Check sheet for the modelled part. Datum: model origin and axes. Units: mm. Face numbers are marked on the shaded views. A direction names the side the tool comes from. Round coordinates to 2 decimals unless told otherwise and drop trailing zeros. Write each loop counter-clockwise with the first axis right and the second up, starting at its lowest first coordinate (ties: lowest second). Pieces come first, ordered by that corner, then holes. Notation, with made-up numbers: (-20.5, 9) -> (26.5, 9) arc R12 cw to (26.5, 32) -> close; hole circle Ø1 at (42.5, 1). An arc over 180 degrees is marked (long way). Put each result on its own line as item: value. Start each with the question number.
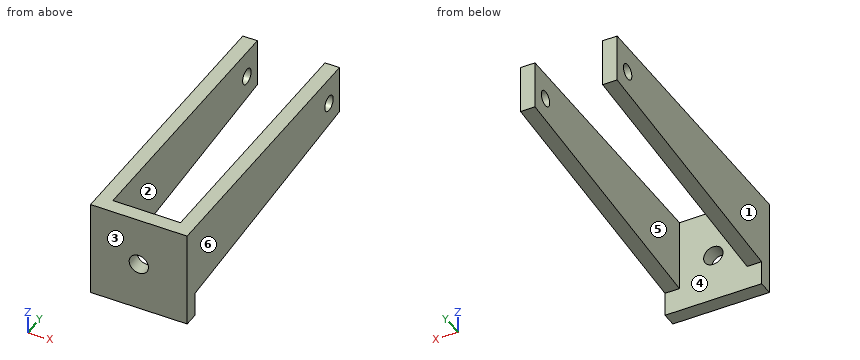
from build123d import *

# Parameters (mm, degrees)
SKETCH_1_W          = 20
SKETCH_1_H          = 20
EXTRUDE_1_DEPTH     = 3
EXTRUDE_2_DEPTH     = 3
EXTRUDE_3_DEPTH     = 3
SKETCH_6_R          = 1.6
CUT_EXTRUDE_1_DEPTH = 21
SKETCH_8_R          = 2
CUT_EXTRUDE_2_DEPTH = 4


with BuildPart() as part:
    # 草图1 → 凸台-拉伸1 (new body)
    with BuildSketch(Plane(origin=(0, 0, 0), x_dir=(1, 0, 0), z_dir=(0, 1, 0))):
        Rectangle(SKETCH_1_W, SKETCH_1_H)
    extrude(amount=EXTRUDE_1_DEPTH)

    # 草图4 → 凸台-拉伸2 (add)
    with BuildSketch(Plane.ZY.offset(10)):
        Polygon((10, 3), (10, 58), (0, 58), (-5, 3), align=None)
    extrude(amount=-EXTRUDE_2_DEPTH)

    # 草图5 → 凸台-拉伸3 (add)
    with BuildSketch(Plane(origin=(10, 0, 0), x_dir=(0, 0, -1), z_dir=(1, 0, 0))):
        Polygon((-10, 3), (5, 3), (0, 58), (-10, 58), align=None)
    extrude(amount=-EXTRUDE_3_DEPTH)

    # 草图6 → 切除-拉伸1 (cut, through all)
    with BuildSketch(Plane(origin=(10, 0, 0), x_dir=(0, 0, -1), z_dir=(1, 0, 0))):
        with Locations((-4.5, 54)):
            Circle(SKETCH_6_R)
    extrude(amount=-CUT_EXTRUDE_1_DEPTH, mode=Mode.SUBTRACT)

    # 草图8 → 切除-拉伸2 (cut, through all)
    with BuildSketch(Plane(origin=(0, 3, 0), x_dir=(1, 0, 0), z_dir=(0, 1, 0))):
        Circle(SKETCH_8_R)
    extrude(amount=-CUT_EXTRUDE_2_DEPTH, mode=Mode.SUBTRACT)


solid = part.part
1. Section check B-B, the plane y = 22.5. Enter the section's corners in (x, z), then the cut area to 3 significant figures.
2. Section check A-A, the plane x = 0. Enter the section's corners in (y, z), then the cut area to 3 significant figures.
3. Draft check along X on the marked faces 3, 4, 5 and 6. Enter one of: released by +X, released by -X, zero draft, split by the parting line, or undercut.
4. Gauge pin test, flat end, axial feed: P1, Ø1.5, axis at x = -1, z = 5, coming from the +Y side. Record the tip position at first contact, or that the pin passes through.
5. Access from +Z, -Z, +X, -X, +Y, -Y to the whole of each face (thin tool, end or side, straight path). Record for the marked faces 1 and 2.
6. Section check D-D, the plane x = -8. Enter the section's corners in (y, z).
7. Section check C-C, the plane z = -3.25. Enter the section's corners in (x, y), then the cut area to 4 significant figures.
8. Material ranges on L1, parallel to X at y = 1, z = 0; L2, parallel to Y at x = 7.6, z = 4.5; L3, parallel to X at y = 45.5, z = 9, recorded low to high. Write a range as [from, to].
Reply:
1. outline: (-10, -3.23) -> (-7, -3.23) -> (-7, 10) -> (-10, 10) -> close; (7, -3.23) -> (10, -3.23) -> (10, 10) -> (7, 10) -> close
1. area: 79.4 mm2
2. outline: (0, -10) -> (3, -10) -> (3, -2) -> (0, -2) -> close; (0, 2) -> (3, 2) -> (3, 10) -> (0, 10) -> close
2. area: 48.0 mm2
3. face 3: zero draft
3. face 4: undercut
3. face 5: undercut
3. face 6: released by +X
4. P1: stops at y = 3
5. face 1: +Z, -Z, -X, +Y, -Y
5. face 2: +Z, -Z, +Y
6. outline: (0, -10) -> (3, -10) -> (3, -5) -> (58, 0) -> (58, 10) -> (0, 10) -> close; hole circle Ø3.2 at (54, 4.5)
7. outline: (-10, 0) -> (10, 0) -> (10, 22.25) -> (7, 22.25) -> (7, 3) -> (-7, 3) -> (-7, 22.25) -> (-10, 22.25) -> close
7. area: 175.5 mm2
8. L1: x = [-10, -2], [2, 10]
8. L2: y = [0, 52.4], [55.6, 58]
8. L3: x = [-10, -7], [7, 10]
